Work out the finished part from the listing and answer in its coordinate system (mm). A direction names the side the tool comes from. Coordinates: 2 decimals unless noted, no trailing zeros. Loops run counter-clockwise (first coordinate to the right, second up) from the corner with the lowest first, then second, coordinate; pieces in that order, holes last. Notation, with made-up numbers: (7, 61) -> (47, 61) arc R17 ccw to (47, 67) -> close; hole circle Ø2 at (-29.5, -13.75). An arc over 180 degrees is marked (long way). One line per question, with ' | ' between items.
```python
from build123d import *

# Parameters (mm, degrees)
SKETCH1_W           = 10
SKETCH1_H           = 10
BOSS_EXTRUDE1_DEPTH = 20
SKETCH2_R           = 1.5
CUT_EXTRUDE1_DEPTH  = 20


with BuildPart() as part:
    # Sketch1 → Boss-Extrude1 (new body)
    with BuildSketch(Plane.XY):
        Rectangle(SKETCH1_W, SKETCH1_H)
        Polygon((2, -1.5), (-2, -1.5), (-2, 1.5), (2, 1.5), (2, 1), (3.5, 1), (3.5, -1), (2, -1), align=None, mode=Mode.SUBTRACT)
    extrude(amount=BOSS_EXTRUDE1_DEPTH)

    # Sketch2 → Cut-Extrude1 (cut)
    with BuildSketch(Plane.XZ.offset(5)):
        with Locations((0, 15)):
            Circle(SKETCH2_R)
    extrude(amount=-CUT_EXTRUDE1_DEPTH, mode=Mode.SUBTRACT)


solid = part.part
```
1) Find section D-D (z = 15). Write down the section's boundary in (x, y), plus the area to 3 significant figures.
Check values:
outline: (-5, -5) -> (-1.5, -5) -> (-1.5, -1.5) -> (-2, -1.5) -> (-2, 1.5) -> (-1.5, 1.5) -> (-1.5, 5) -> (-5, 5) -> close; (1.5, -5) -> (5, -5) -> (5, 5) -> (1.5, 5) -> (1.5, 1.5) -> (2, 1.5) -> (2, 1) -> (3.5, 1) -> (3.5, -1) -> (2, -1) -> (2, -1.5) -> (1.5, -1.5) -> close | area: 64.0 mm^2
2) Find section A-A (z = 3). Write down the section's boundary in (x, y).
Check values:
outline: (-5, -5) -> (5, -5) -> (5, 5) -> (-5, 5) -> close; hole (-2, -1.5) -> (2, -1.5) -> (2, -1) -> (3.5, -1) -> (3.5, 1) -> (2, 1) -> (2, 1.5) -> (-2, 1.5) -> close
3) Find the intervals of material crossed by line 1 along Y through (x, z) = (0.75, 19); line 2 along Z through (x, y) = (0, 3.9); line 3 along Y through (x, z) = (2.25, 12), in increasing order.
Check values:
line 1: y = -5 to -1.5, 1.5 to 5 | line 2: z = 0 to 13.5, 16.5 to 20 | line 3: y = -5 to -1, 1 to 5
4) For faces 1 (the face through (3, 1, 10)), 2 (the face through (-5, 0, 10)), determine the directions among +Z, -Z, +X, -X, +Y, -Y from which every point of the face is accessible in a straight line to the end or side of a thin tool.
Check values:
face 1: +Z, -Z | face 2: +Z, -Z, -X, +Y, -Y
5) The mould has two halves that part along X. Classify faces 3 (the face through (-1.11, -3.27, 16.01)), 4 (the face through (-2.3, 0.1, 0)), 5 (the face through (5, 0, 10)), 6 (the face through (-1.11, 3.23, 16.01)): released by +X, released by -X, zero draft, split by the parting line, or undercut.
Check values:
face 3: undercut | face 4: zero draft | face 5: released by +X | face 6: undercut
6) Find section B-B (x = 2.25). Write down the section's boundary in (y, z).
Check values:
outline: (-5, 0) -> (-1, 0) -> (-1, 20) -> (-5, 20) -> close; (1, 0) -> (5, 0) -> (5, 20) -> (1, 20) -> close
7) A flat-ended cylindrical pin translates along its axis: pin 1 (2.5 mm diameter, centred on x = 0, z = 15, fed in from -Y). Find the tip coordinate at first contact, or state that the pin passes through.
Check values:
pin 1: passes through
8) Find section C-C (y = -3.5). Write down the section's boundary in (x, z).
Check values:
outline: (-5, 0) -> (5, 0) -> (5, 20) -> (-5, 20) -> close; hole circle Ø3 at (0, 15)
